Geometry: final body of the model. Coordinates: model frame, mm. A direction names the side the tool comes from. Give positions to 0.01 mm unless a question says otherwise; leave off trailing zeros.
Autodesk Inventor part; units mm, degrees
ref_plane "Work Plane4" through (0, 100, 0) normal (0, 0.7071068, 0.7071068) x (1, 0, 0)
ref_plane "YZ Plane" through (0, 0, 0) normal (1, 0, 0) x (0, 1, 0)
ref_plane "XZ Plane" through (0, 0, 0) normal (0, 1, 0) x (-1, 0, 0)
sketch "Sketch1" plane through (0, 0, 0) normal (0, 0, 1) x (1, 0, 0)
  arc A0 (12.7973, -6.8176) -> (-12.597, -7.1809) centre (0, 0) ccw
  arc A1 (50.4829, -6.2785) -> (26.2017, -6.6259) centre (38.25, 0) ccw
  arc A2 (85.5853, -5.7763) -> (63.5844, -6.091) centre (74.5, 0) ccw
  arc A3 (117.8988, -5.314) -> (98.5072, -5.5914) centre (108.125, 0) ccw
  arc A4 (147.9764, -4.8837) -> (130.6669, -5.1313) centre (139.25, 0) ccw
  arc A5 (177.1345, -4.4665) -> (160.4967, -4.7045) centre (168.75, 0) ccw
  line L0 (-20, 20) -> (188.75, 20)
  line L1 (188.75, 20) -> (188.75, -4.3003)
  line L2 (-20, 20) -> (-20, -7.2868)
  line L3 (-20, -7.2868) -> (188.75, -4.3003)
  dimension "d0" = 29
  dimension "d1" = 27.5
  dimension "d2" = 25
  dimension "d3" = 22.25
  dimension "d4" = 20
  dimension "d5" = 19
  dimension "d6" = 38.25
  dimension "d7" = 36.25
  dimension "d8" = 33.625
  dimension "d9" = 31.125
  dimension "d10" = 29.5
  dimension "d11" = 0
  dimension "d12" = 0
  dimension "d13" = 0
  dimension "d14" = 0
  dimension "d15" = 0
  dimension "d20" = 20
  dimension "d22" = 20
  dimension "d23" = 20
  dimension "d24" = 7
  dimension "d25" = 4.586
sketch "Sketch4" plane through (0, 0, 0) normal (1, 0, 0) x (0, 1, 0)
  line L0 (0, 0) -> (29.9033, -29.9033)
  line L1 (0, 5.9807) -> (0, -35.884)
  point P0 (100, 0)
  dimension "d51" = 45
  dimension "d53" = 0
  dimension "d55" = 29.9033
  dimension "d98" = 100
ref_plane "Work Plane4" through (0, 100, 0) normal (0, 0.7071068, 0.7071068) x (1, 0, 0)
ref_plane "Work Plane3" through (-10, 0, 0) normal (0, 0.7071068, 0.7071068) x (1, 0, 0)
sketch "Sketch5" plane through (-10, 0, 0) normal (0, 0.7071068, 0.7071068) x (1, 0, 0)
  arc A0 (39.5473, 0.4692) -> (14.153, 0.1059) centre (26.75, 7.2868) ccw
  arc A1 (69.4829, 1.0084) -> (45.2017, 0.661) centre (57.25, 7.2868) ccw
  arc A2 (96.8353, 1.5106) -> (74.8344, 1.1958) centre (85.75, 7.2868) ccw
  arc A3 (121.3988, 1.9729) -> (102.0072, 1.6954) centre (111.625, 7.2868) ccw
  arc A4 (143.7264, 2.4032) -> (126.4169, 2.1555) centre (135, 7.2868) ccw
  arc A5 (165.1345, 2.8203) -> (148.4967, 2.5823) centre (156.75, 7.2868) ccw
  line L0 (10, 27.2868) -> (168.5, 27.2868)
  line L1 (168.5, 27.2868) -> (168.5, 2.9865)
  line L2 (10, 27.2868) -> (10, 0)
  line L3 (10, 0) -> (14.153, 0.1059)
  line L4 (39.5473, 0.4692) -> (45.2017, 0.661)
  line L5 (69.4829, 1.0084) -> (74.8344, 1.1958)
  line L6 (96.8353, 1.5106) -> (102.0072, 1.6954)
  line L7 (165.1345, 2.8203) -> (168.5, 2.9865)
  line L8 (121.3988, 1.9729) -> (126.4169, 2.1555)
  line L9 (143.7264, 2.4032) -> (148.4967, 2.5823)
  dimension "d56" = 29
  dimension "d57" = 27.5
  dimension "d58" = 25
  dimension "d59" = 22.25
  dimension "d60" = 20
  dimension "d61" = 19
  dimension "d62" = 30.5
  dimension "d63" = 28.5
  dimension "d64" = 25.875
  dimension "d65" = 23.375
  dimension "d66" = 21.75
  dimension "d67" = 0
  dimension "d68" = 0
  dimension "d69" = 0
  dimension "d70" = 0
  dimension "d71" = 0
  dimension "d72" = 20
  dimension "d73" = 11.75
  dimension "d74" = 16.75
sketch "Sketch6" plane through (0, 100, 0) normal (0, 0.7071068, 0.7071068) x (1, 0, 0)
  arc A0 (29.5473, 0.4692) -> (4.153, 0.1059) centre (16.75, 7.2868) ccw
  arc A1 (59.4829, 1.0084) -> (35.2017, 0.661) centre (47.25, 7.2868) ccw
  arc A2 (86.8353, 1.5106) -> (64.8344, 1.1958) centre (75.75, 7.2868) ccw
  arc A3 (111.3988, 1.9729) -> (92.0072, 1.6954) centre (101.625, 7.2868) ccw
  arc A4 (133.7264, 2.4032) -> (116.4169, 2.1555) centre (125, 7.2868) ccw
  arc A5 (155.1345, 2.8203) -> (138.4967, 2.5823) centre (146.75, 7.2868) ccw
  line L0 (0, 27.2868) -> (158.5, 27.2868)
  line L1 (158.5, 27.2868) -> (158.5, 2.9865)
  line L2 (0, 27.2868) -> (0, 0)
  line L3 (0, 0) -> (4.153, 0.1059)
  line L4 (29.5473, 0.4692) -> (35.2017, 0.661)
  line L5 (59.4829, 1.0084) -> (64.8344, 1.1958)
  line L6 (86.8353, 1.5106) -> (92.0072, 1.6954)
  line L7 (111.3988, 1.9729) -> (116.4169, 2.1555)
  line L8 (133.7264, 2.4032) -> (138.4967, 2.5823)
  line L9 (155.1345, 2.8203) -> (158.5, 2.9865)
  point P0 (0, -70.7107)
  dimension "d77" = 29
  dimension "d78" = 27.5
  dimension "d79" = 25
  dimension "d80" = 22.25
  dimension "d81" = 20
  dimension "d82" = 19
  dimension "d83" = 30.5
  dimension "d84" = 28.5
  dimension "d85" = 25.875
  dimension "d86" = 23.375
  dimension "d87" = 21.75
  dimension "d88" = 0
  dimension "d89" = 0
  dimension "d90" = 0
  dimension "d91" = 0
  dimension "d92" = 0
  dimension "d93" = 20
  dimension "d94" = 11.75
  dimension "d95" = 16.75
loft "Loft1" add profiles "Sketch6", "Sketch5"
sketch "Sketch7" plane through (0, 0, 0) normal (0, 1, 0) x (-1, 0, 0)
  line L0 (0, 0) -> (0, -19.2947)
  line L1 (0, -19.2947) -> (-158.5, -19.2947)
  line L2 (-158.5, -19.2947) -> (-158.5, -2.1118)
  line L3 (-158.5, -2.1118) -> (-155.1345, -1.9943)
  ellipse E0 centre (-146.75, -5.1526) end of major axis (-156.25, -5.1526) minor radius 6.7175 (-155.1345, -1.9943) -> (-138.4967, -1.826) ccw
  line L4 (-138.4967, -1.826) -> (-133.7264, -1.6993)
  ellipse E1 centre (-125, -5.1526) end of major axis (-135, -5.1526) minor radius 7.0711 (-133.7264, -1.6993) -> (-116.4169, -1.5242) ccw
  line L5 (-116.4169, -1.5242) -> (-111.3988, -1.395)
  ellipse E2 centre (-101.625, -5.1526) end of major axis (-112.75, -5.1526) minor radius 7.8666 (-111.3988, -1.395) -> (-92.0072, -1.1989) ccw
  line L6 (-92.0072, -1.1989) -> (-86.8353, -1.0681)
  ellipse E3 centre (-75.75, -5.1526) end of major axis (-88.25, -5.1526) minor radius 8.8388 (-86.8353, -1.0681) -> (-64.8344, -0.8456) ccw
  line L7 (-64.8344, -0.8456) -> (-59.4829, -0.713)
  ellipse E4 centre (-47.25, -5.1526) end of major axis (-61, -5.1526) minor radius 9.7227 (-59.4829, -0.713) -> (-35.2017, -0.4674) ccw
  line L8 (-35.2017, -0.4674) -> (-29.5473, -0.3318)
  ellipse E5 centre (-16.75, -5.1526) end of major axis (-31.25, -5.1526) minor radius 10.253 (-29.5473, -0.3318) -> (-4.153, -0.0749) ccw
  line L9 (-4.153, -0.0749) -> (0, 0)
  line L10 (0, 0) -> (0, -19.2947)
  line L11 (0, -19.2947) -> (-158.5, -19.2947)
  line L12 (-158.5, -19.2947) -> (-158.5, -2.1118)
  line L13 (-158.5, -2.1118) -> (0, 0)
  point P0 (0, 0)
sketch "Sketch10" plane through (0, 19.2947, -19.2947) normal (-1, 0, 0) x (0, 0, 1)
  line L0 (19.2947, 80.7053) -> (0, 100)
  line L1 (0, 100) -> (0, 0)
  line L2 (19.2947, -19.2947) -> (0, 0)
  line L3 (19.2947, 80.7053) -> (19.2947, -19.2947)
  line L4 (19.2947, -19.2947) -> (19.2947, -24.2947)
  line L5 (0, 0) -> (0, -22.6066)
  line L6 (0, -22.6066) -> (19.2947, -24.2947)
  line L7 (0, -22.6066) -> (-24.9049, -20.4278)
  line L8 (-24.9049, -20.4278) -> (0, 17.5461)
  line L9 (0, 100) -> (0, 0)
  line L10 (0, 17.5461) -> (0, 0)
  point P0 (19.2947, -19.2947)
  dimension "d106" = 5
  dimension "d111" = 85
  dimension "d113" = 25
  dimension "d114" = 40
sketch "Sketch11" plane through (158.5, 2.1118, -2.1118) normal (1, 0, 0) x (0, 0, -1)
  line L0 (17.1829, 117.1829) -> (0, 100)
  line L1 (0, 100) -> (0, 0)
  line L2 (17.1829, 17.1829) -> (0, 0)
  line L3 (17.1829, 117.1829) -> (17.1829, 17.1829)
  line L4 (17.1829, 17.1829) -> (0, 0)
  line L5 (10.1119, 10.1119) -> (-0.5876, -0.5876)
  line L6 (17.1829, -5.4237) -> (-2.1118, -7.1118)
  line L7 (0, 0) -> (0, -6.927)
  line L8 (17.1829, -5.4237) -> (0, -6.927)
  line L9 (17.1829, -5.4237) -> (17.1829, 17.1829)
  line L10 (0, -6.927) -> (17.1829, -5.4237)
  line L11 (17.1829, -5.4237) -> (42.0878, -3.2448)
  line L12 (42.0878, -3.2448) -> (17.1829, 34.5763)
  line L13 (17.1829, 117.1829) -> (17.1829, 17.1829)
  line L14 (17.1829, 17.1829) -> (17.1829, 34.5763)
  point P0 (-2.1118, -2.1118)
  point P1 (17.1829, -7.1118)
  point P2 (-0.4125, -0.4125)
  dimension "d115" = 25
  dimension "d116" = 40
loft "Loft3" add profiles "Sketch10", "Sketch11" contours L4 L6 L5 L2 | L1 L5 L7 L8 / L12 L11 L9 L3 | L2 L9 L6 L7
properties part number "coin_holder"
Item 1: Reachability of faces 1 (the face through (80, 77, -19.295)), 2 (the face through (82, 115, -15)) from +Z, -Z, +X, -X, +Y, -Y: full face, straight path, thin tool, end or side. Return the list, or none.
Found:
face 1: -Z, +X, -X, +Y
face 2: +Z, +X, -X, +Y
Item 2: Line query: L1, parallel to Z at x = 64.5, y = 39; L2, parallel to Y at x = 44.5, z = -5; L3, parallel to Y at x = 24.5, z = -18. Output: solid intervals per line, ascending.
Found:
L1: z = -19.29 to -9.01, -1.3 to -0.84
L2: y = -4.56 to 5
L3: y = -3.43 to 118
Item 3: Pin query (flat end, axial travel): pin 1 Ø12 at (x, z) = (82, -38) entering from +Y; pin 2 Ø12 at (x, z) = (37, -16.5) entering from -Y; pin 3 Ø1 at (x, y) = (89, 35.5) entering from +Z; pin 4 Ø8 at (y, z) = (71, -22) entering from -X. Return the tip coordinate at first contact, or that it passes through.
Found:
pin 1: stops at y = 17.43
pin 2: stops at y = -4.08
pin 3: stops at z = -1.11
pin 4: stops at x = 0
